```python
from build123d import *

# Parameters (mm, degrees)
F0_W      = 431.8
F0_H      = 254
F1_DEPTH  = 355.6
F2_W      = 419.5426851511
F2_H      = 345.1122520491
F3_DEPTH  = 246.38
F5_R      = 25.4
F6_DEPTH  = 20.066
F7_W      = 352.0536348224
F7_H      = 66.7818960792
F8_DEPTH  = 431.801
F9_W      = 44.8005609214
F9_H      = 10.6667876244
F10_DEPTH = 254.001


# Not quite as in the source:
# - a feature names something its author has since deleted; it is built from what else it names


with BuildPart() as f1:
    # F0 (on Front) → F1 (new body)
    with BuildSketch(Plane.XZ):
        Rectangle(F0_W, F0_H)
    extrude(amount=F1_DEPTH)

    # F2 (on face) → F3 (cut)
    with BuildSketch(Plane.XY.offset(127)):
        with Locations((1.86265e-05, -177.8631941415)):
            Rectangle(F2_W, F2_H)
    extrude(amount=-F3_DEPTH, mode=Mode.SUBTRACT)

    # F5 (on face) → F6 (join)
    with BuildSketch(Plane.XZ.offset(355.6)):
        with Locations((0, 70.3678135578)):
            Circle(F5_R)
    extrude(amount=F6_DEPTH)

    # F7 (on face) → F8 (cut, through all)
    with BuildSketch(Plane.YZ.offset(215.9)):
        with Locations((-176.0268174112, 93.6090519604)):
            Rectangle(F7_W, F7_H)
    extrude(amount=-F8_DEPTH, mode=Mode.SUBTRACT)

    # F9 (on face) → F10 (cut, through all)
    with BuildSketch(Plane.XY.offset(127)):
        with Locations((-0.0037699938, -367.3357367516)):
            Rectangle(F9_W, F9_H)
    extrude(amount=-F10_DEPTH, mode=Mode.SUBTRACT)


solid = f1.part
```
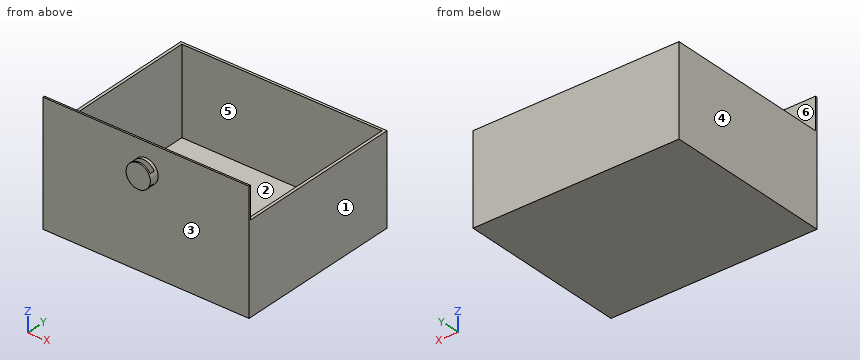
The listing builds one solid part. Answer for the finished solid, in the listing's coordinates (mm). Face numbers are marked on the shaded views. A direction names the side the tool comes from. Round coordinates to 2 decimals unless told otherwise and drop trailing zeros. Write each loop counter-clockwise with the first axis right and the second up, starting at its lowest first coordinate (ties: lowest second). Pieces come first, ordered by that corner, then holes. Notation, with made-up numbers: (-32.5, 86) -> (-10.5, 86) arc R14 ccw to (-10.5, 108) -> close; hole circle Ø5 at (47, 5). An arc over 180 degrees is marked (long way). Answer as a JSON object with one key per item and string values. Group by question number.
Q1. Which of the six approach directions +Z, -Z, +X, -X, +Y, -Y give full straight-line access (tool end or side, diameter ignored) to the marked faces 4, 5 and 6?
Q2. Section C-C (y = -253) is taken. Write down the section's boundary in (x, z).
Q3. Section A-A (x = 0) is taken. Write down the section's boundary in (y, z), plus the area to 3 significant figures.
Q4. Determine the mould class of the marked faces 1, 2 and 3 for opening direction Y: pulls with the +Y half, pulls with the -Y half, needs draft (parallel to the pull), parting line crosses it, or undercut.
Q5. Section B-B (z = -24.5) is taken. Write down the section's boundary in (x, y), plus the area to 3 significant figures.
Q6. Section D-D (x = 119.5) is taken. Write down the section's boundary in (y, z).
Q7. Straight lines are drawn through the part: line 1 along X through (y, z) = (-214, -65); line 2 along Y through (x, z) = (98, 44); line 3 along Z through (x, y) = (169, -99.5). For each, find the intervals that lie inside material, in ascending order.
Q8. Each of these flat-tipped pins is pushed along its axis until it touches: pin 1 Ø10 at (x, z) = (-168.5, 69.5) entering from -Y; pin 2 Ø11.5 at (y, z) = (-368.5, 74.5) entering from -X; pin 3 Ø12 at (x, y) = (99, -329) entering from +Z. Where does it stop, or does it pass through?
Check values:
{
 "1": {"face 4": "+Z, -Z, -X, +Y, -Y", "face 5": "+Z", "face 6": "+Z, +X, -X, +Y"},
 "2": {"outline": "(-215.9, -127) -> (215.9, -127) -> (215.9, 60.22) -> (209.77, 60.22) -> (209.77, -119.38) -> (-209.77, -119.38) -> (-209.77, 60.22) -> (-215.9, 60.22) -> close"},
 "3": {"outline": "(-375.67, 44.97) -> (-372.67, 44.97) -> (-372.67, 95.77) -> (-375.67, 95.77) -> close; (-362, 44.97) -> (-355.6, 44.97) -> (-355.6, -127) -> (0, -127) -> (0, 60.22) -> (-5.31, 60.22) -> (-5.31, -119.38) -> (-350.42, -119.38) -> (-350.42, 60.22) -> (-352.05, 60.22) -> (-352.05, 127) -> (-355.6, 127) -> (-355.6, 95.77) -> (-362, 95.77) -> close", "area": "5,310 mm^2"},
 "4": {"face 1": "needs draft", "face 2": "undercut", "face 3": "pulls with the -Y half"},
 "5": {"outline": "(-215.9, -355.6) -> (215.9, -355.6) -> (215.9, 0) -> (-215.9, 0) -> close; hole (-209.77, -350.42) -> (209.77, -350.42) -> (209.77, -5.31) -> (-209.77, -5.31) -> close", "area": "8,760 mm^2"},
 "6": {"outline": "(-355.6, -127) -> (0, -127) -> (0, 60.22) -> (-5.31, 60.22) -> (-5.31, -119.38) -> (-350.42, -119.38) -> (-350.42, 60.22) -> (-352.05, 60.22) -> (-352.05, 127) -> (-355.6, 127) -> close"},
 "7": {"line 1": "-215.9 to -209.77, 209.77 to 215.9", "line 2": "-355.6 to -350.42, -5.31 to 0", "line 3": "-127 to -119.38"},
 "8": {"pin 1": "y = -355.6", "pin 2": "x = -25.4", "pin 3": "z = -119.38"}
}
